Build history of the part. All positions in model axes, mm. Round coordinates to 2 decimals unless told otherwise and drop trailing zeros. Write each loop counter-clockwise with the first axis right and the second up, starting at its lowest first coordinate (ties: lowest second). Pieces come first, ordered by that corner, then holes. Notation, with made-up numbers: M 32.25,68.25 L 42.25,68.25 A30 ccw 42.25,93.25 Z; hole C -4,-27.5 d5. An arc over 180 degrees is marked long. One line per item, written item: value. Start each with the question number.
```python
from build123d import *

# Parameters (mm, degrees)
BOSS_EXTRUDE1_DEPTH                 = 2
F_3_1_3_1_DIAMETER_HOLE1_AT_2_COUNT = 2
F_3_1_3_1_DIAMETER_HOLE1_AT_2_PITCH = 28
F_3_1_3_1_DIAMETER_HOLE1_AT_3_COUNT = 2
F_3_1_3_1_DIAMETER_HOLE1_AT_3_PITCH = 57.306195128
F_3_1_3_1_DIAMETER_HOLE1_AT_4_COUNT = 2
F_3_1_3_1_DIAMETER_HOLE1_AT_4_PITCH = 50
F_3_1_3_1_DIAMETER_HOLE1_AT_5_COUNT = 2
F_3_1_3_1_DIAMETER_HOLE1_AT_5_PITCH = 16
F_3_1_3_1_DIAMETER_HOLE1_AT_6_COUNT = 2
F_3_1_3_1_DIAMETER_HOLE1_AT_6_PITCH = 32.249030993


with BuildPart() as part:
    # Sketch1 → Boss-Extrude1 (new body)
    with BuildSketch(Plane(origin=(0, 0, 0), x_dir=(1, 0, 0), z_dir=(0, 1, 0))):
        with BuildLine():
            Line((22, -19), (-22, -19))
            ThreePointArc((-22, -19), (-27.656854249, -16.656854249), (-30, -11))
            Line((-30, -11), (-30, 11))
            ThreePointArc((-30, 11), (-27.656854249, 16.656854249), (-22, 19))
            Line((-22, 19), (22, 19))
            ThreePointArc((22, 19), (27.656854249, 16.656854249), (30, 11))
            Line((30, 11), (30, -11))
            ThreePointArc((30, -11), (27.656854249, -16.656854249), (22, -19))
        make_face()
    extrude(amount=BOSS_EXTRUDE1_DEPTH)

    # Hole → Ø3.1 (3.1) Diameter Hole1 (revolve, cut)
    with BuildSketch(Plane(origin=(25, 2, -14), x_dir=(0, 0, 1), z_dir=(1, 0, 0))):
        Polygon((0, 0), (0, 2), (1.55, 2), (1.55, 1.7), (3.25, 0), align=None)
    f_3_1_3_1_diameter_hole1 = revolve(axis=Axis((25, 8.35, -14), (0, -1, 0)), mode=Mode.SUBTRACT)

    # Ø3.1 (3.1) Diameter Hole1 at 2: Ø3.1 (3.1) Diameter Hole1 ×2
    with Locations(*[(0, 0, i * F_3_1_3_1_DIAMETER_HOLE1_AT_2_PITCH) for i in range(1, F_3_1_3_1_DIAMETER_HOLE1_AT_2_COUNT)]):
        add(f_3_1_3_1_diameter_hole1, mode=Mode.SUBTRACT)

    # Ø3.1 (3.1) Diameter Hole1 at 3: Ø3.1 (3.1) Diameter Hole1 ×2
    with Locations(*[Vector(-0.872506016, 0, 0.488603369) * (i * F_3_1_3_1_DIAMETER_HOLE1_AT_3_PITCH) for i in range(1, F_3_1_3_1_DIAMETER_HOLE1_AT_3_COUNT)]):
        add(f_3_1_3_1_diameter_hole1, mode=Mode.SUBTRACT)

    # Ø3.1 (3.1) Diameter Hole1 at 4: Ø3.1 (3.1) Diameter Hole1 ×2
    with Locations(*[(-i * F_3_1_3_1_DIAMETER_HOLE1_AT_4_PITCH, 0, 0) for i in range(1, F_3_1_3_1_DIAMETER_HOLE1_AT_4_COUNT)]):
        add(f_3_1_3_1_diameter_hole1, mode=Mode.SUBTRACT)

    # Ø3.1 (3.1) Diameter Hole1 at 5: Ø3.1 (3.1) Diameter Hole1 ×2
    with Locations(*[(-i * F_3_1_3_1_DIAMETER_HOLE1_AT_5_PITCH, 0, 0) for i in range(1, F_3_1_3_1_DIAMETER_HOLE1_AT_5_COUNT)]):
        add(f_3_1_3_1_diameter_hole1, mode=Mode.SUBTRACT)

    # Ø3.1 (3.1) Diameter Hole1 at 6: Ø3.1 (3.1) Diameter Hole1 ×2
    with Locations(*[Vector(-0.496138938, 0, 0.868243142) * (i * F_3_1_3_1_DIAMETER_HOLE1_AT_6_PITCH) for i in range(1, F_3_1_3_1_DIAMETER_HOLE1_AT_6_COUNT)]):
        add(f_3_1_3_1_diameter_hole1, mode=Mode.SUBTRACT)


solid = part.part
```
Item 1: Cut at B-B, the plane z = 14. Write the cut outline in (x, y), plus the area to 3 significant figures.
Item 2: Cut at C-C, the plane y = 0.85. Write the cut outline in (x, z), plus the area to 3 significant figures.
Item 3: Drop flat-ended pins along their axis: pin 1 (2.5 mm diameter, centred on x = -25, z = 14, fed in from +Y); pin 2 (4 mm diameter, centred on x = 25, z = 14, fed in from +Y); pin 3 (5 mm diameter, centred on x = -25, z = -14, fed in from +Y); pin 4 (5 mm diameter, centred on x = -0.5, z = -12.5, fed in from -Y). Give the stop position or say it passes through.
Item 4: Cut at D-D, the plane x = -25. Write the cut outline in (y, z), plus the area to 3 significant figures.
Item 5: Drill centre lines: line 1 (Z direction, x = 7.5, y = 0.9); line 2 (Z direction, x = 25, y = 0.15); line 3 (X direction, y = 0.2, z = -14). Where is each one in solid material? Low to high.
Item 6: Cut at A-A, the plane x = 9. Write the cut outline in (y, z), plus the area to 3 significant figures.
Computed values:
1. outline: M -29.42,0 L -26.55,0 L -26.55,0.3 L -28.25,2 L -29.42,2 Z; M -23.45,0 L 7.45,0 L 7.45,0.3 L 5.75,2 L -21.75,2 L -23.45,0.3 Z; M 10.55,0 L 23.45,0 L 23.45,0.3 L 21.75,2 L 12.25,2 L 10.55,0.3 Z; M 26.55,0 L 29.42,0 L 29.42,2 L 28.25,2 L 26.55,0.3 Z
1. area: 90.4 mm2
2. outline: M -30,-11 A8 ccw -22,-19 L 22,-19 A8 ccw 30,-11 L 30,11 A8 ccw 22,19 L -22,19 A8 ccw -30,11 Z; hole C -25,-14 d4.2; hole C -25,14 d4.2; hole C 9,-14 d4.2; hole C 9,14 d4.2; hole C 25,-14 d4.2; hole C 25,14 d4.2
2. area: 2,140 mm2
3. pin 1: passes through
3. pin 2: stops at y = 0.75
3. pin 3: stops at y = 1.25
3. pin 4: stops at y = 0
4. outline: M 0,-18.42 L 2,-18.42 L 2,-17.25 L 0.3,-15.55 L 0,-15.55 Z; M 0,-12.45 L 0.3,-12.45 L 2,-10.75 L 2,10.75 L 0.3,12.45 L 0,12.45 Z; M 0,15.55 L 0.3,15.55 L 2,17.25 L 2,18.42 L 0,18.42 Z
4. area: 55.5 mm2
5. line 1: z = -19 to -15.54, -12.46 to 12.46, 15.54 to 19
5. line 2: z = -18.42 to -15.55, -12.45 to 12.45, 15.55 to 18.42
5. line 3: x = -29.42 to -26.55, -23.45 to 7.45, 10.55 to 23.45, 26.55 to 29.42
6. outline: M 0,-19 L 2,-19 L 2,-17.25 L 0.3,-15.55 L 0,-15.55 Z; M 0,-12.45 L 0.3,-12.45 L 2,-10.75 L 2,10.75 L 0.3,12.45 L 0,12.45 Z; M 0,15.55 L 0.3,15.55 L 2,17.25 L 2,19 L 0,19 Z
6. area: 57.8 mm2
